Autodesk Inventor part; units mm, degrees
ref_plane "Плоскость YZ" through (0, 0, 0) normal (1, 0, 0) x (0, 1, 0)
ref_plane "Плоскость XZ" through (0, 0, 0) normal (0, 1, 0) x (-1, 0, 0)
ref_plane "Плоскость XY" through (0, 0, 0) normal (0, 0, 1) x (1, 0, 0)
sketch "Эскиз1" plane through (0, 0, 0) normal (0, 1, 0) x (-1, 0, 0)
  line L0 (10.9667, 22.3) -> (-10.9667, 22.3)
  line L1 (-10.9667, 22.3) -> (-10.9667, -22.3)
  line L2 (-10.9667, -22.3) -> (10.9667, -22.3)
  line L3 (10.9667, -22.3) -> (10.9667, 22.3)
  line L4 (10.9667, 22.3) -> (-10.9667, -22.3) construction
  line L5 (-10.9667, 22.3) -> (10.9667, -22.3) construction
  point P0 (0, 0)
  dimension "d0" = 44.6
  dimension "d1" = 21.9333
extrude "Выдавливание1" add sketch "Эскиз1" along normal blind 3.58
fillet "Сопряжение1" radius 0.5 12 edges at (0, 3.58, 22.3) (0, 0, 22.3) (10.9667, 1.79, 22.3) (-10.9667, 1.79, 22.3) (-10.9667, 3.58, 0) (10.9667, 3.58, 0) (10.9667, 0, 0) (-10.9667, 0, 0) (0, 3.58, -22.3) (0, 0, -22.3) (-10.9667, 1.79, -22.3) (10.9667, 1.79, -22.3)
sketch "Эскиз2" plane through (0, 3.58, 0) normal (0, 1, 0) x (1, 0, 0)
  line L0 (-2.1, 24.4) -> (2.1, 24.4)
  line L1 (2.1, 24.4) -> (2.1, 20.2)
  line L2 (2.1, 20.2) -> (-2.1, 20.2)
  line L3 (-2.1, 20.2) -> (-2.1, 24.4)
  line L4 (10.4667, 22.3) -> (-10.4667, 22.3)
  line L5 (-2.1, 24.4) -> (2.1, 20.2) construction
  line L6 (2.1, 24.4) -> (-2.1, 20.2) construction
  point P0 (0, 0)
  point P1 (0, 22.3)
  dimension "d5" = 4.2
  dimension "d6" = 4.2
extrude "Выдавливание2" cut sketch "Эскиз2" against normal blind 10
mirror "Зеркальное отражение1" about plane through (0, 0, 0) normal (0, 0, 1) of "Выдавливание2"
properties part number "Test2" material "Типовой"
Part model, mm, in its own coordinate system. A direction names the side the tool comes from. Give positions to 0.01 mm unless a question says otherwise; leave off trailing zeros. Loops run counter-clockwise (first coordinate to the right, second up) from the corner with the lowest first, then second, coordinate; pieces in that order, holes last. Notation, with made-up numbers: (-14.5, -24.5) -> (44.5, -24.5) arc R6 cw to (44.5, -13.5) -> close; hole circle Ø3 at (40, -20.5). An arc over 180 degrees is marked (long way). Write each question's results on one line, items separated by ' | '. Start each with the question number.
Q1. Wall check: L1, parallel to Z at x = 0.5, y = 0.4; L2, parallel to Z at x = 6.75, y = 3.3. Give the ranges that are in metal, low to high.
Q2. Band-saw the part on B-B on x = -1.25. List the corners of the cut face in (y, z), plus the area to 3 significant figures.
Q3. Which spindle directions (+Z, -Z, +X, -X, +Y, -Y) get a long thin tool onto all of the face, cutting with end or side? Do faces 1 (the face through (-2.1, 2, -21)), 2 (the face through (-2.1, 2, 21)), 3 (the face through (-6, 2, 22.3)). Say none if no direction does.
Q4. Band-saw the part on A-A on y = 1.7. List the corners of the cut face in (x, z).
Results are:
1) L1: z = -20.2 to 20.2 | L2: z = -22.25 to 22.25
2) outline: (0, -20.2) -> (3.58, -20.2) -> (3.58, 20.2) -> (0, 20.2) -> close | area: 145 mm²
3) face 1: -Z, +Y, -Y | face 2: +Z, +Y, -Y | face 3: +Z, +X, -X, +Y, -Y
4) outline: (-10.97, -21.8) arc R0.5 ccw to (-10.47, -22.3) -> (-2.1, -22.3) -> (-2.1, -20.2) -> (2.1, -20.2) -> (2.1, -22.3) -> (10.47, -22.3) arc R0.5 ccw to (10.97, -21.8) -> (10.97, 21.8) arc R0.5 ccw to (10.47, 22.3) -> (2.1, 22.3) -> (2.1, 20.2) -> (-2.1, 20.2) -> (-2.1, 22.3) -> (-10.47, 22.3) arc R0.5 ccw to (-10.97, 21.8) -> close
